Verification items for the finished model (mm, model axes). Face numbers are marked on the shaded views. A direction names the side the tool comes from. Coordinates: 2 decimals unless noted, no trailing zeros. Order: outer loops, then holes, each group sorted by start corner. A loop starts at its lowest first (then second) coordinate and runs counter-clockwise, first axis right, second up. Notation, with made-up numbers: (73.25, -27.75) - (90.25, -27.75) arc R30 ccw to (90.25, -4.75) - close; hole circle Ø2 at (54, 59.5). An arc over 180 degrees is marked (long way). Answer as CSV lines item,"result". Start each with the question number.
1. Section check C-C (z = 3.5). Record the cut outline in (x, y), and give its area (3 significant figures).
2. Section check B-B (x = 0). Record the cut outline in (y, z) (3 decimals), and give its area (3 significant figures).
3. Material ranges on L1, parallel to Z at x = 0.25, y = 1.25; L2, parallel to Z at x = -1.5, y = -2.75; L3, parallel to Y at x = 0, z = -4.25 (3 decimals), recorded low to high. Write a range as [from, to].
4. Section check A-A (z = -0.25). Record the cut outline in (x, y) (3 decimals), and give its area (3 significant figures).
5. Set-up check for the marked faces 1, 2 and 3: record each of +Z, -Z, +X, -X, +Y, -Y from which the full face is reachable in a straight line by a thin tool's end or side.
6. Go/stop test with flat-tipped pins: pin 1 (0.7 mm diameter, centred on y = 1, z = -2.5, fed in from -X); pin 2 (0.6 mm diameter, centred on x = -1.5, z = 5.5, fed in from +Y) (3 decimals); pin 3 (1.5 mm diameter, centred on y = 0, z = -2, fed in from +X). Record where each tip stops, or that it passes through.
7. Mould release check, pull along Y, two halves, no side actions. Record for the marked faces 4, 5 and 6: pulls with the +Y half, pulls with the -Y half, needs draft (parallel to the pull), parting line crosses it, or undercut.
Autodesk Inventor part; units mm, degrees
ref_plane "YZ Plane" through (0, 0, 0) normal (1, 0, 0) x (0, 1, 0)
ref_plane "XZ Plane" through (0, 0, 0) normal (0, 1, 0) x (-1, 0, 0)
ref_plane "XY Plane" through (0, 0, 0) normal (0, 0, 1) x (1, 0, 0)
sketch "Sketch1" plane through (0, 0, 0) normal (0, 0, 1) x (1, 0, 0)
  circle A0 centre (0, 0) radius 2.8
  line L0 (-0.675, 0.675) -> (-0.675, 2.025)
  line L1 (-0.675, 2.025) -> (0.675, 2.025)
  line L2 (0.675, 2.025) -> (0.675, 0.675)
  line L3 (0.675, 0.675) -> (2.025, 0.675)
  line L4 (2.025, 0.675) -> (2.025, -0.675)
  line L5 (2.025, -0.675) -> (0.675, -0.675)
  line L6 (0.675, -0.675) -> (0.675, -2.025)
  line L7 (0.675, -2.025) -> (-0.675, -2.025)
  line L8 (-0.675, -2.025) -> (-0.675, -0.675)
  line L9 (-0.675, -0.675) -> (-2.025, -0.675)
  line L10 (-2.025, -0.675) -> (-2.025, 0.675)
  line L11 (-2.025, 0.675) -> (-0.675, 0.675)
  circle A1 centre (0, 0) radius 4.94 construction
  circle A2 centre (0, 0) radius 4.47
  point P0 (-6.07, -6.1)
  dimension "d16" = 9.88
  dimension "d17" = 0.47
extrude "Extrusion8" add sketch "Sketch1" along normal blind 5 contours A0 | L0 L1 L2 L3 L4 L5 L6 L7 L8 L9 L10 L11 | A2
extrude "Extrusion9" add sketch "Sketch1" against normal blind 4.8 contours A0
sketch "Sketch4" plane through (0, 0, 5) normal (0, 0, 1) x (1, 0, 0)
  line L0 (-3.616, 1.525) -> (3.616, 1.525) construction
  line L1 (3.616, 1.525) -> (3.616, -1.525) construction
  line L2 (3.616, -1.525) -> (-3.616, -1.525) construction
  line L3 (-3.616, -1.525) -> (-3.616, 1.525) construction
  line L4 (0.6327, 1.525) -> (-0.1384, -1.525)
  line L5 (-0.1384, -1.525) -> (-0.9788, -1.525)
  line L6 (-0.9788, -1.525) -> (-1.4682, 0.3609)
  line L7 (-1.4682, 0.3609) -> (-1.9402, -1.525)
  line L8 (-1.9402, -1.525) -> (-2.7831, -1.525)
  line L9 (-2.7831, -1.525) -> (-3.5542, 1.525)
  line L10 (-3.5542, 1.525) -> (-2.7583, 1.525)
  line L11 (-2.7583, 1.525) -> (-2.3382, -0.5166)
  line L12 (-2.3382, -0.5166) -> (-1.829, 1.525)
  line L13 (-1.829, 1.525) -> (-1.0677, 1.525)
  line L14 (-1.0677, 1.525) -> (-0.5833, -0.519)
  line L15 (-0.5833, -0.519) -> (-0.1434, 1.525)
  line L16 (-0.1434, 1.525) -> (0.6327, 1.525)
  line L17 (3.5913, -1.525) -> (2.7064, -1.525)
  line L18 (2.7064, -1.525) -> (2.1182, -0.5536)
  line L19 (2.1182, -0.5536) -> (1.5176, -1.525)
  line L20 (1.5176, -1.525) -> (0.6698, -1.525)
  line L21 (0.6698, -1.525) -> (1.6609, 0.0099)
  line L22 (1.6609, 0.0099) -> (0.7094, 1.525)
  line L23 (0.7094, 1.525) -> (1.5942, 1.525)
  line L24 (1.5942, 1.525) -> (2.1454, 0.6031)
  line L25 (2.1454, 0.6031) -> (2.7114, 1.525)
  line L26 (2.7114, 1.525) -> (3.5592, 1.525)
  line L27 (3.5592, 1.525) -> (2.6026, 0.042)
  line L28 (2.6026, 0.042) -> (3.5913, -1.525)
  point P0 (0, 0)
  point P1 (0, -1.525)
  point P2 (3.616, 0)
  point P3 (0, 0)
  point P4 (0, 0)
extrude "Extrusion10" add sketch "Sketch4" along normal blind 0.9
properties part number "IPC WX key"
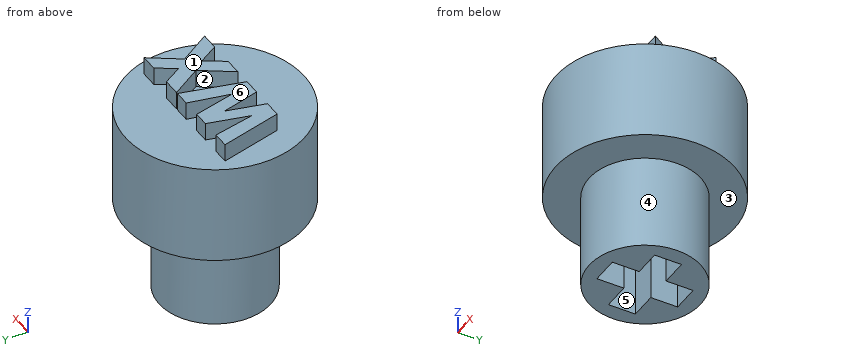
Evaluation:
1,outline,"circle Ø8.94 at (0, 0)"
1,area,"62.8 mm²"
2,outline,"(-4.47, 0) - (-2.8, 0) - (-2.8, -4.8) - (-2.025, -4.8) - (-2.025, 0) - (2.025, 0) - (2.025, -4.8) - (2.8, -4.8) - (2.8, 0) - (4.47, 0) - (4.47, 5) - (1.525, 5) - (1.525, 5.9) - (-0.978, 5.9) - (-0.978, 5) - (-4.47, 5) - close"
2,area,"54.4 mm²"
3,L1,"z = [0, 5.9]"
3,L2,"z = [0, 5]"
3,L3,"y = [-2.8, -2.025], [2.025, 2.8]"
4,outline,"circle Ø5.6 at (0, 0); hole (-2.025, -0.675) - (-0.675, -0.675) - (-0.675, -2.025) - (0.675, -2.025) - (0.675, -0.675) - (2.025, -0.675) - (2.025, 0.675) - (0.675, 0.675) - (0.675, 2.025) - (-0.675, 2.025) - (-0.675, 0.675) - (-2.025, 0.675) - close"
4,area,"15.5 mm²"
5,face 1,"+Z, +X, -X, +Y, -Y"
5,face 2,"+Z"
5,face 3,"-Z"
6,pin 1,"stops at x = -2.72"
6,pin 2,"stops at y = 1.525"
6,pin 3,"stops at x = 2.8"
7,face 4,"parting line crosses it"
7,face 5,"undercut"
7,face 6,"needs draft"
